Could you check a few things on this model? Use its own coordinates, in mm. A direction names the side the tool comes from. Coordinates: 2 decimals unless noted, no trailing zeros. Order: outer loops, then holes, each group sorted by start corner. A loop starts at its lowest first (then second) coordinate and runs counter-clockwise, first axis right, second up. Notation, with made-up numbers: (-33.75, 51) -> (-23.75, 51) arc R23 ccw to (-23.75, 89) -> close; hole circle Ø9 at (30, -8.5). An arc over 180 degrees is marked (long way). Use a Markdown table: item, result. Add a question column.
1) If we section it at C-C (y = -15.25): Write out the boundary of the cut face in (x, z), plus the area to 3 significant figures.
2) If we section it at B-B (x = -5): Write out the boundary of the cut face in (y, z).
3) Which directions (+Z, -Z, +X, -X, +Y, -Y) give clear straight access to the entire face, cutting with the end or side of a thin tool? Please do faces 1 (the flat face through (-33, 0, -2)), 2 (the flat face through (-34.03, -1.32, -2.24)), 3 (the flat face through (1, -11, -1.5)).
4) If I drill on L1, parallel to X at y = -7, z = -4; L2, parallel to Y at x = -43.5, z = -2.5, over which ranges is the centre line in solid material (lowest first)? Write a range as [from, to].
5) Will this pin go through, and if not, where does the flat tip stop? pin 1 Ø0.7 at (x, y) = (0.5, -9) entering from +Z.
```python
from build123d import *

# Parameters (mm, degrees)
F0_W      = 10
F0_H      = 10
F1_DEPTH  = 2
F3_DEPTH  = 60
F5_DEPTH  = 2
F7_DEPTH  = 2
F9_SIZE   = 1
F10_R     = 5.08
F11_DEPTH = 2.9920059478
F12_DEPTH = 10
F13_DEPTH = 10
F14_DEPTH = 10
F16_DEPTH = 2
F17_SIZE  = 1.99999
F18_R     = 1


# Not quite as in the source:
# - a fillet or chamfer is up to 0.001 mm smaller than in the source, because OpenCascade refuses the exact size


with BuildPart() as f1:
    # F0 (on Right) → F1 (new body)
    with BuildSketch(Plane.YZ):
        with Locations((-5, -5)):
            Rectangle(F0_W, F0_H)
    extrude(amount=F1_DEPTH)

    # F2 (on face) → F3 (join)
    with BuildSketch(Plane.YZ.offset(2)):
        Polygon((0, -3), (0, 0), (-2.5980762114, -1.5), align=None)
    extrude(amount=-F3_DEPTH)

    # F4 (on face) → F5 (cut, through all)
    with BuildSketch(Plane(origin=(0, 0, 0), x_dir=(0, -1, 0), z_dir=(-1, 0, 0))):
        Polygon((10, 0), (0, 0), (2.5980762114, -1.5), align=None)
    extrude(amount=-F5_DEPTH, mode=Mode.SUBTRACT)

    # F6 (on face) → F7 (cut, through all)
    with BuildSketch(Plane.YZ.offset(2)):
        Polygon((-10, -1.5), (-2.5980762114, -1.5), (-10, 0), align=None)
    extrude(amount=-F7_DEPTH, mode=Mode.SUBTRACT)

    # F9
    f9_edges = [f1.edges().sort_by_distance(p)[0] for p in [
        (0, -1.299038, -2.25),
    ]]
    chamfer(f9_edges, length=F9_SIZE)

    # F10
    f10_edges = [f1.edges().sort_by_distance(p)[0] for p in [
        (1, -2.598076, -1.5),
    ]]
    fillet(f10_edges, radius=F10_R)

    # F8 (on face) → F11 (cut, through all)
    with BuildSketch(Plane.YZ.offset(2)):
        Polygon((0, -10), (0, -3.0103854369), (-8.4680961445, -10), align=None)
    extrude(amount=-F11_DEPTH, mode=Mode.SUBTRACT)

    # F12 (add): a face of the model
    f12_faces = [f1.faces().sort_by_distance(p)[0] for p in [
        (-58, -0.8660254038, -1.5),
    ]]
    extrude(f12_faces, amount=F12_DEPTH)

    # F13 (add): a face of the model
    f13_faces = [f1.faces().sort_by_distance(p)[0] for p in [
        (1, -10, -5.75),
    ]]
    extrude(f13_faces, amount=F13_DEPTH)

    # F14 (add): a face of the model
    f14_faces = [f1.faces().sort_by_distance(p)[0] for p in [
        (1, -14.2340480722, -10),
    ]]
    extrude(f14_faces, amount=F14_DEPTH)

    # F15 (on face) → F16 (cut, through all)
    with BuildSketch(Plane.YZ.offset(2)):
        Polygon((-8.4680961445, -20), (-8.4680961445, -10), (-20, -20), align=None)
    extrude(amount=-F16_DEPTH, mode=Mode.SUBTRACT)

    # F17 (size 2 in the source; OpenCascade refuses exactly that, so slightly less here)
    f17_edges = [f1.edges().sort_by_distance(p)[0] for p in [
        (0, -20, -10.75),
    ]]
    chamfer(f17_edges, length=F17_SIZE)

    # F18
    f18_edges = [f1.edges().sort_by_distance(p)[0] for p in [
        (0.999995, -19.000005, -1.5),
        (0.999995, -19.000005, -19.132845),
    ]]
    fillet(f18_edges, radius=F18_R)


solid = f1.part
```
Answer sheet:
| question | item | result |
|---|---|---|
| 1 | outline | (0, -15.88) -> (2, -15.88) -> (2, -1.5) -> (0, -1.5) -> close |
| 1 | area | 28.8 mm2 |
| 2 | outline | (-2.6, -1.5) -> (0, -3) -> (0, 0) -> close |
| 3 | face 1 | +Z, -Z, +X, -X, +Y |
| 3 | face 2 | -Z, -X, -Y |
| 3 | face 3 | +Z, +X, -X, -Y |
| 4 | L1 | [0, 2] |
| 4 | L2 | [-0.87, 0] |
| 5 | pin 1 | z = -1.5 |
